```python
from build123d import *

# Parameters (mm, degrees)
SKETCH_W     = 160
SKETCH_H     = 370
PAD_DEPTH    = 18
SKETCH001_W  = 60
SKETCH001_H  = 18
POCKET_DEPTH = 12
CHAMFER_SIZE = 15
FILLET_R     = 10


with BuildPart() as part:
    # Sketch → Pad (new body)
    with BuildSketch(Plane.XY):
        Rectangle(SKETCH_W, SKETCH_H)
    extrude(amount=PAD_DEPTH)

    # Sketch001 → Pocket (cut)
    with BuildSketch(Plane.XY.offset(18)):
        with Locations((0, 111)):
            Rectangle(SKETCH001_W, SKETCH001_H)
    pocket = extrude(amount=-POCKET_DEPTH, mode=Mode.SUBTRACT)

    # Mirrored: Pocket across Sketch001 H_Axis
    add(pocket.mirror(Plane(origin=(0, 0, 18), x_dir=(0, 0, 1), z_dir=(0, 1, 0))), mode=Mode.SUBTRACT)

    # Chamfer
    chamfer_edges = [part.edges().sort_by_distance(p)[0] for p in [
        (-80, -185, 9),
        (-80, 185, 9),
        (80, 185, 9),
        (80, -185, 9),
    ]]
    chamfer(chamfer_edges, length=CHAMFER_SIZE)

    # Fillet
    fillet_edges = [part.edges().sort_by_distance(p)[0] for p in [
        (65, -185, 9),
        (80, -170, 9),
        (-65, -185, 9),
        (-80, -170, 9),
        (-80, 170, 9),
        (-65, 185, 9),
        (65, 185, 9),
        (80, 170, 9),
    ]]
    fillet(fillet_edges, radius=FILLET_R)


solid = part.part
```
Here's how the part is built. I have some questions about the finished solid (model axes, mm). A direction names the side the tool comes from. Round coordinates to 2 decimals unless told otherwise and drop trailing zeros. Order: outer loops, then holes, each group sorted by start corner. A loop starts at its lowest first (then second) coordinate and runs counter-clockwise, first axis right, second up. Notation, with made-up numbers: (12, 13.5) -> (32, 13.5) arc R24 ccw to (32, 39.5) -> close; hole circle Ø1 at (42, 31). An arc over 180 degrees is marked (long way). Use a Markdown table: item, result. Add a question column.
(1) I need wall thicknesses on line 1 along Y through (x, z) = (16, 15.5); line 2 along X through (y, z) = (119.5, 13.25); line 3 along Z through (x, y) = (12.5, 112). Which ranges of each line are inside material? Lowest first, please.
(2) For pin 1 Ø9 at (x, y) = (10, 107.5) entering from +Z, with a flat end and sliding along its axis, tell me the tip position at first contact or that it passes through.
(3) Suppose I cut it at B-B, the plane x = -1. Please give me the cut outline in (y, z).
(4) If we mould it in two halves opening along Y, with no side actions, what happens to faces 3 (the face through (-30, -111, 12)), 4 (the face through (-80, -2, 9)), 5 (the face through (-64.735, 184.218, 9.126)), 6 (the face through (79.218, -169.735, 9.126))? For each: released by +Y, released by -Y, zero draft, split by the parting line, or undercut.
(5) Suppose I cut it at A-A, the plane z = 12.5. Please give me the cut outline in (x, y).
(6) For faces 1 (the face through (-1, 185, 9)), 2 (the face through (0, 120, 12)), which set-ups out of +Z, -Z, +X, -X, +Y, -Y let a thin tool reach every point of the face, with its end or its side?
Verdict:
| question | item | result |
|---|---|---|
| 1 | line 1 | -185 to -120, -102 to 102, 120 to 185 |
| 1 | line 2 | -80 to -30, 30 to 80 |
| 1 | line 3 | 0 to 6 |
| 2 | pin 1 | z = 6 |
| 3 | outline | (-185, 0) -> (185, 0) -> (185, 18) -> (120, 18) -> (120, 6) -> (102, 6) -> (102, 18) -> (-102, 18) -> (-102, 6) -> (-120, 6) -> (-120, 18) -> (-185, 18) -> close |
| 4 | face 3 | undercut |
| 4 | face 4 | zero draft |
| 4 | face 5 | released by +Y |
| 4 | face 6 | released by -Y |
| 5 | outline | (-80, -165.86) arc R10 ccw to (-77.07, -172.93) -> (-67.93, -182.07) arc R10 ccw to (-60.86, -185) -> (60.86, -185) arc R10 ccw to (67.93, -182.07) -> (77.07, -172.93) arc R10 ccw to (80, -165.86) -> (80, 165.86) arc R10 ccw to (77.07, 172.93) -> (67.93, 182.07) arc R10 ccw to (60.86, 185) -> (-60.86, 185) arc R10 ccw to (-67.93, 182.07) -> (-77.07, 172.93) arc R10 ccw to (-80, 165.86) -> close; hole (-30, -120) -> (30, -120) -> (30, -102) -> (-30, -102) -> close; hole (-30, 102) -> (30, 102) -> (30, 120) -> (-30, 120) -> close |
| 6 | face 1 | +Z, -Z, +X, -X, +Y |
| 6 | face 2 | +Z |
